```python
from build123d import *

# Parameters (mm, degrees)
EXTRUDE_THIN1_DEPTH = 762
FILLET1_R           = 1.016


with BuildPart() as part:
    # Sketch1 → Extrude-Thin1 (new body)
    with BuildSketch(Plane.XY):
        Polygon((0, 0), (-15.875, 0), (-15.875, -12.7), (-44.45, -12.7), (-44.45, 1.5875), (-41.275, 1.5875), (-41.275, 49.2125), (-44.45, 49.2125), (-44.45, 63.5), (-15.875, 63.5), (-15.875, 50.8), (0, 50.8), (0, 49.784), (-16.891, 49.784), (-16.891, 62.484), (-43.434, 62.484), (-43.434, 50.2285), (-40.259, 50.2285), (-40.259, 0.5715), (-43.434, 0.5715), (-43.434, -11.684), (-16.891, -11.684), (-16.891, 1.016), (0, 1.016), align=None)
    extrude(amount=-EXTRUDE_THIN1_DEPTH)

    # Fillet1
    fillet1_edges = [part.edges().sort_by_distance(p)[0] for p in [
        (-16.891, 49.784, -381),
        (-40.259, 50.2285, -381),
        (-40.259, 0.5715, -381),
        (-16.891, 1.016, -381),
        (-15.875, -12.7, -381),
        (-44.45, -12.7, -381),
        (-44.45, 1.5875, -381),
        (-44.45, 49.2125, -381),
        (-44.45, 63.5, -381),
        (-15.875, 63.5, -381),
    ]]
    fillet(fillet1_edges, radius=FILLET1_R)


solid = part.part
```
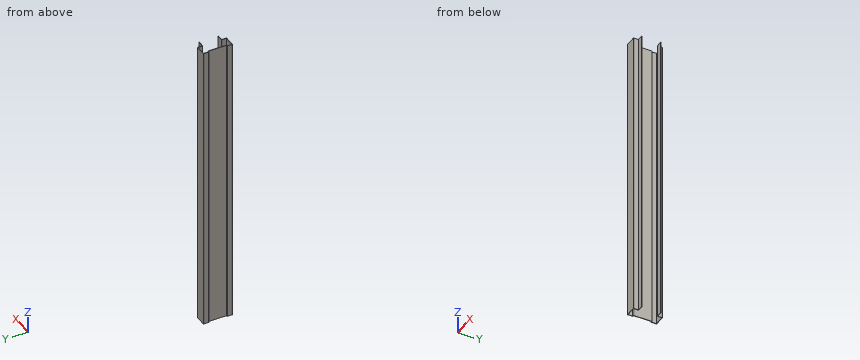
Read the model definition and answer for the solid it produces. Units are mm, in the model's axes. Give positions to 0.01 mm unless a question says otherwise; leave off trailing zeros. Loops run counter-clockwise (first coordinate to the right, second up) from the corner with the lowest first, then second, coordinate; pieces in that order, holes last.
Item 1: The part is cut by section C-C (y = 22). Write down the section's boundary in (x, z) (3 decimals).
Item 2: Each of these flat-tipped pins is pushed along its axis until it touches: pin 1 Ø8 at (x, z) = (-8.5, -470.5) entering from -Y; pin 2 Ø24 at (y, z) = (35, -466) entering from -X (3 decimals); pin 3 Ø12 at (x, y) = (-20, 2.5) entering from +Z; pin 4 Ø3.5 at (y, z) = (57.5, -535) entering from +X (3 decimals). Where does it stop, or does it pass through?
Item 3: Find the intervals of material crossed by line 1 along Y through (x, z) = (-33, -639); line 2 along Y through (x, z) = (-11.5, -89); line 3 along X through (y, z) = (50.5, -580.5), in increasing order.
Item 4: The part is cut by section A-A (x = -27). Write down the section's boundary in (y, z).
Taken from the geometry:
1. outline: (-41.275, -762) - (-40.259, -762) - (-40.259, 0) - (-41.275, 0) - close
2. pin 1: stops at y = 0
2. pin 2: stops at x = -41.275
2. pin 3: stops at z = 0
2. pin 4: stops at x = -15.875
3. line 1: y = -12.7 to -11.68, 62.48 to 63.5
3. line 2: y = 0 to 1.02, 49.78 to 50.8
3. line 3: x = -44.45 to -43.43, -16.85 to 0
4. outline: (-12.7, -762) - (-11.68, -762) - (-11.68, 0) - (-12.7, 0) - close; (62.48, -762) - (63.5, -762) - (63.5, 0) - (62.48, 0) - close
